from build123d import *

# Parameters (mm, degrees)
EXTRUDE_1728_DEPTH   = 2.5
EXTRUDE_1728_2_DEPTH = 2.5
SKETCH_3_W           = 4.096784854
SKETCH_3_H           = 4.817676116
SKETCH_3_R           = 1.2
EXTRUDE_1_DEPTH      = 2
EXTRUDE_2_REACH      = 41.086
SKETCH_5_W           = 2.5
SKETCH_5_H           = 2.5


with BuildPart() as part:
    # Sketch 2 → Extrude 1728 (new body)
    with BuildSketch(Plane(origin=(0, 0, 0), x_dir=(1, 0, 0), z_dir=(0, 1, 0))):
        Polygon((11.136061282, -24.056246494), (20.323880385, -24.056246494), (20.323880385, -15.656749138), (17.100927376, -15.656749138), (14.000927376, -15.656749138), (10.862052049, -15.656749138), (9.6, -15.656749138), (9.6, -22.156749138), (11.073569208, -22.156749138), align=None)
        with BuildLine():
            Line((14.000927376, -19.227513168), (14.000927376, -22.422888537))
            ThreePointArc((14.000927376, -22.422888537), (14.03898761, -22.614230253), (14.147373985, -22.776441927))
            Line((14.147373985, -22.776441927), (15.162186301, -23.791254243))
            ThreePointArc((15.162186301, -23.791254243), (15.515739691, -23.937700852), (15.869293082, -23.791254243))
            Line((15.869293082, -23.791254243), (16.954480766, -22.706066558))
            ThreePointArc((16.954480766, -22.706066558), (17.062867142, -22.543854884), (17.100927376, -22.352513168))
            Line((17.100927376, -22.352513168), (17.100927376, -19.297888537))
            ThreePointArc((17.100927376, -19.297888537), (17.062867142, -19.10654682), (16.954480766, -18.944335146))
            Line((16.954480766, -18.944335146), (15.869293082, -17.859147462))
            ThreePointArc((15.869293082, -17.859147462), (15.515739691, -17.712700852), (15.162186301, -17.859147462))
            Line((15.162186301, -17.859147462), (14.147373985, -18.873959777))
            ThreePointArc((14.147373985, -18.873959777), (14.03898761, -19.036171452), (14.000927376, -19.227513168))
        make_face(mode=Mode.SUBTRACT)
    extrude(amount=EXTRUDE_1728_DEPTH)



with BuildPart() as body_2:
    # Sketch 2 → Extrude 1728 2 (new body)
    with BuildSketch(Plane(origin=(0, 0, 0), x_dir=(1, 0, 0), z_dir=(0, 1, 0))):
        Polygon((-11.136061282, -24.056246494), (-20.323880385, -24.056246494), (-20.323880385, -15.656749138), (-17.100927376, -15.656749138), (-14.000927376, -15.656749138), (-10.862052049, -15.656749138), (-9.6, -15.656749138), (-9.6, -22.156749138), (-11.073569208, -22.156749138), align=None)
        with BuildLine():
            Line((-14.000927376, -19.227513168), (-14.000927376, -22.422888537))
            ThreePointArc((-14.000927376, -22.422888537), (-14.03898761, -22.614230253), (-14.147373985, -22.776441927))
            Line((-14.147373985, -22.776441927), (-15.162186301, -23.791254243))
            ThreePointArc((-15.162186301, -23.791254243), (-15.515739691, -23.937700852), (-15.869293082, -23.791254243))
            Line((-15.869293082, -23.791254243), (-16.954480766, -22.706066558))
            ThreePointArc((-16.954480766, -22.706066558), (-17.062867142, -22.543854884), (-17.100927376, -22.352513168))
            Line((-17.100927376, -22.352513168), (-17.100927376, -19.297888537))
            ThreePointArc((-17.100927376, -19.297888537), (-17.062867142, -19.10654682), (-16.954480766, -18.944335146))
            Line((-16.954480766, -18.944335146), (-15.869293082, -17.859147462))
            ThreePointArc((-15.869293082, -17.859147462), (-15.515739691, -17.712700852), (-15.162186301, -17.859147462))
            Line((-15.162186301, -17.859147462), (-14.147373985, -18.873959777))
            ThreePointArc((-14.147373985, -18.873959777), (-14.03898761, -19.036171452), (-14.000927376, -19.227513168))
        make_face(mode=Mode.SUBTRACT)
    extrude(amount=EXTRUDE_1728_2_DEPTH)


with BuildPart() as part_1:
    add(part.part)

    add(body_2.part)  # Extrude 1 merges body 2
    # Sketch 3 → Extrude 1 (add)
    # profile 1 of 2: a face of its own
    with BuildSketch(Plane(origin=(0, 0, 15.656749138), x_dir=(-1, 0, 0), z_dir=(0, 0, -1))):
        with Locations((-11.648392427, 4.908838058)):
            Rectangle(SKETCH_3_W, SKETCH_3_H)
        with Locations((-11.5, 5)):
            Circle(SKETCH_3_R, mode=Mode.SUBTRACT)
    # profile 2 of 2: a face of its own
    with BuildSketch(Plane(origin=(0, 0, 15.656749138), x_dir=(-1, 0, 0), z_dir=(0, 0, -1))):
        with Locations((11.648392427, 4.908838058)):
            Rectangle(SKETCH_3_W, SKETCH_3_H)
        with Locations(Location((11.5, 5, 0), (0, 0, 180))):
            Circle(SKETCH_3_R, mode=Mode.SUBTRACT)
    extrude(amount=-EXTRUDE_1_DEPTH)

    # Sketch 5 → Extrude 2 (add, up to next)
    with BuildSketch(Plane.ZY.offset(-9.6), mode=Mode.PRIVATE) as extrude_2_sk1:
        with Locations((20.906749138, 1.25)):
            Rectangle(SKETCH_5_W, SKETCH_5_H)
    extrude_2_tool1 = extrude(extrude_2_sk1.sketch, amount=EXTRUDE_2_REACH, mode=Mode.PRIVATE) - part_1.part
    add(extrude_2_tool1.solids().sort_by_distance((9.6, 1.25, 20.906749))[0])


solid = part_1.part
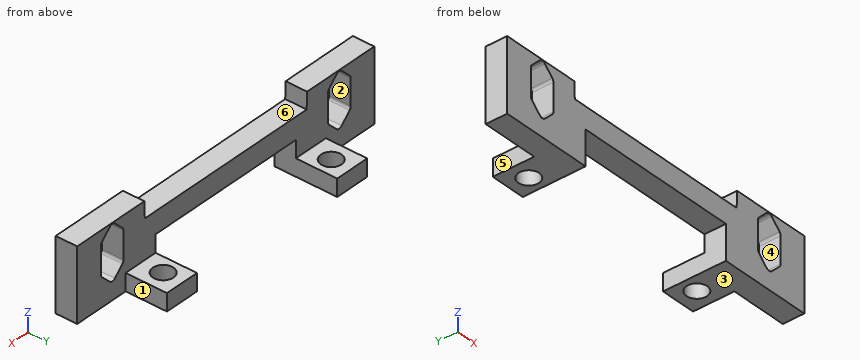
The listing builds one solid part. Answer for the finished solid, in the listing's coordinates (mm). Face numbers are marked on the shaded views. A direction names the side the tool comes from. Coordinates: 2 decimals unless noted, no trailing zeros. Order: outer loops, then holes, each group sorted by start corner. A loop starts at its lowest first (then second) coordinate and runs counter-clockwise, first axis right, second up. Notation, with made-up numbers: (-29.5, 9) -> (-9.5, 9) arc R12 cw to (-9.5, 13) -> close; hole circle Ø2 at (40.25, 20). An arc over 180 degrees is marked (long way). Answer in a Markdown table with one row per item. Add a question column.
Item 1: Find section A-A (z = 21). Write down the section's boundary in (x, y).
Item 2: Each of these flat-tipped pins is pushed along its axis until it touches: P1, Ø3, axis at x = 11.5, y = 5, coming from the -Z side; P2, Ø2, axis at x = -11.5, y = 5, coming from the +Z side; P3, Ø2, axis at x = 11, y = 5.5, coming from the +Z side; P4, Ø2, axis at x = -1, y = 1.5, coming from the -Z side. Where does it stop, or does it pass through?
Item 3: Find section D-D (y = 5). Write down the section's boundary in (x, z).
Item 4: Find section B-B (x = 11.5). Write down the section's boundary in (y, z), then the cut area to 3 significant figures.
Item 5: Find section C-C (y = 3). Write down the section's boundary in (x, z), then the cut area to 3 significant figures.
Item 6: Find the intervals of material crossed by L1, parallel to X at y = 1.25, z = 22; L2, parallel to Y at x = -11.5, z = 16.1; L3, parallel to X at y = 6.75, z = 17.5, in increasing order. Write a range as from..to.
Item 7: Determine the mould class of the marked faces 1, 2 and 3 for opening direction X: +X half, -X half, draft (parallel to the pull), parting line (faces both ways), or undercut.
Item 8: Which of the six approach directions +Z, -Z, +X, -X, +Y, -Y give full straight-line access (tool end or side, diameter ignored) to the marked faces 4, 5 and 6?
Result set:
| question | item | result |
|---|---|---|
| 1 | outline | (-20.32, 0) -> (-17.1, 0) -> (-17.1, 2.5) -> (-20.32, 2.5) -> close; (-14, 0) -> (14, 0) -> (14, 2.5) -> (-14, 2.5) -> close; (17.1, 0) -> (20.32, 0) -> (20.32, 2.5) -> (17.1, 2.5) -> close |
| 2 | P1 | stops at z = 15.66 |
| 2 | P2 | passes through |
| 2 | P3 | stops at z = 17.66 |
| 2 | P4 | stops at z = 19.66 |
| 3 | outline | (-13.7, 15.66) -> (-12.7, 15.66) -> (-12.7, 17.66) -> (-13.7, 17.66) -> close; (-10.3, 15.66) -> (-9.6, 15.66) -> (-9.6, 17.66) -> (-10.3, 17.66) -> close; (9.6, 15.66) -> (10.3, 15.66) -> (10.3, 17.66) -> (9.6, 17.66) -> close; (12.7, 15.66) -> (13.7, 15.66) -> (13.7, 17.66) -> (12.7, 17.66) -> close |
| 4 | outline | (0, 15.66) -> (3.8, 15.66) -> (3.8, 17.66) -> (2.5, 17.66) -> (2.5, 24.06) -> (0, 24.06) -> close; (6.2, 15.66) -> (7.32, 15.66) -> (7.32, 17.66) -> (6.2, 17.66) -> close |
| 4 | area | 25.8 mm² |
| 5 | outline | (-13.7, 15.66) -> (-9.6, 15.66) -> (-9.6, 17.66) -> (-13.7, 17.66) -> close; (9.6, 15.66) -> (13.7, 15.66) -> (13.7, 17.66) -> (9.6, 17.66) -> close |
| 5 | area | 16.4 mm² |
| 6 | L1 | x = -20.32..-17.1, -14..14, 17.1..20.32 |
| 6 | L2 | y = 0..3.8, 6.2..7.32 |
| 6 | L3 | x = -13.7..-9.6, 9.6..13.7 |
| 7 | face 1 | +X half |
| 7 | face 2 | undercut |
| 7 | face 3 | draft |
| 8 | face 4 | +Y, -Y |
| 8 | face 5 | +Z, -Z, -X, +Y |
| 8 | face 6 | +Z, +Y, -Y |
